Model file for the job. Use its own axes, mm. Face numbers are marked on the shaded views. Round coordinates to 2 decimals unless told otherwise and drop trailing zeros. Write each loop counter-clockwise with the first axis right and the second up, starting at its lowest first coordinate (ties: lowest second). Pieces come first, ordered by that corner, then holes. Notation, with made-up numbers: (48.25, -29) - (89.25, -29) arc R22 cw to (89.25, 8) - close; hole circle Ø8 at (-8, 8). An arc over 180 degrees is marked (long way). Answer as a JSON object with one key per item and string values. Group by question number.
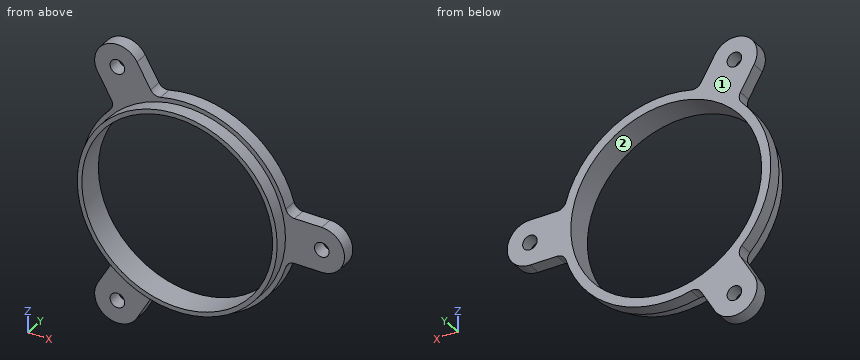
Autodesk Inventor part; units mm, degrees
ref_plane "YZ Plane" through (0, 0, 0) normal (1, 0, 0) x (0, 1, 0)
ref_plane "XZ Plane" through (0, 0, 0) normal (0, 1, 0) x (-1, 0, 0)
ref_plane "XY Plane" through (0, 0, 0) normal (0, 0, 1) x (1, 0, 0)
sketch "Sketch1" plane through (0, 0, 0) normal (0, 0, 1) x (1, 0, 0)
  line L0 (-21, 0) -> (-21, 6)
  line L1 (-21, 6) -> (-23, 6)
  line L2 (-23, 6) -> (-23, 3)
  line L3 (-23, 3) -> (-22, 3)
  line L4 (-22, 3) -> (-22, 0)
  line L5 (-22, 0) -> (-21, 0)
  line L6 (0, -1.2) -> (0, 7.2)
  point P0 (0, 0)
  point P1 (-22, 1.5)
  dimension "d0" = 22
  dimension "d1" = 1
  dimension "d2" = 23
  dimension "d3" = 3
  dimension "d4" = 3
revolve "Revolution1" add sketch "Sketch1" angle 360 about axis through (0, -10, 0) along (0, 1, 0)
sketch "Sketch2" plane through (0, 6, 0) normal (0, 1, 0) x (1, 0, 0)
  circle A0 centre (0, 0) radius 30 construction
  circle A1 centre (30, 0) radius 5
  circle A2 centre (0, 0) radius 23
  line L0 (30, 5) -> (22.4499, 5)
  line L1 (30, -5) -> (22.4499, -5)
  dimension "d6" = 60
  dimension "d7" = 10
extrude "Extrusion1" add sketch "Sketch2" against normal blind 3 contours A1 | A1 L1 A2 L0
fillet "Fillet1" radius 2 2 edges at (22.4499, 4.5, 5) (22.4499, 4.5, -5)
sketch "Sketch3" plane through (30, 6, 0) normal (0, 1, 0) x (1, 0, 0)
  arc A0 (0, -5) -> (0, 5) centre (0, 0) ccw
  point P0 (-30, 0)
hole "Hole1" at (30, 6, 0) direction (0, -1, 0) diameter 3.2 end through all
pattern_circular "Circular Pattern1" count 3 over 360 about axis through (0, 3, 0) along (0, 1, 0) of "Extrusion1", "Hole1", "Fillet1"
properties part number "Electrode-Fixed-Press" material "Brass"
(1) Flat gauge pins, fed straight in: pin 1 (0.9 mm diameter, centred on x = 28.5, y = 4.5, fed in from -Z); pin 2 (1 mm diameter, centred on x = 18.5, y = 3, fed in from +Z); pin 3 (1.5 mm diameter, centred on x = 16, y = 1.5, fed in from +Z); pin 4 (3 mm diameter, centred on x = -15, z = -25.98, fed in from +Y). Where does each tip first touch, or does it go through?
(2) Slice it at D-D (y = 4.9). Write the cut outline in (x, z), then the cut area to 3 significant figures.
(3) Slice it at A-A (x = 0). Write the cut outline in (y, z).
(4) Pull direction X, two halves, no side cores. Call the marked faces 1 and 2: pulls with the +X half, pulls with the -X half, needs draft (parallel to the pull), parting line crosses it, or undercut.
(5) Slice it at B-B (z = 0). Write the cut outline in (x, y), then the cut area to 3 significant figures.
(6) Drill centre lines: line 1 (Z direction, x = 30, y = 5.1); line 2 (X direction, y = 2.2, z = -7.5); line 3 (X direction, y = 0.3, z = 11). Where is each one in solid material? Low to high. Write a range as from..to.
(7) Slice it at C-C (z = 26.5). Write the cut outline in (x, y), then the cut area to 3 significant figures.
Answer:
{
 "1": {"pin 1": "z = -5", "pin 2": "z = 14.32", "pin 3": "z = 15.86", "pin 4": "through"},
 "2": {"outline": "(-19.33, -23.48) arc R5 ccw to (-10.67, -28.48) - (-7.67, -23.28) arc R2 cw to (-5.46, -22.34) arc R23 ccw to (22.08, -6.44) arc R2 cw to (24, -5) - (30, -5) arc R5 ccw to (30, 5) - (24, 5) arc R2 cw to (22.08, 6.44) arc R23 ccw to (-5.46, 22.34) arc R2 cw to (-7.67, 23.28) - (-10.67, 28.48) arc R5 ccw to (-19.33, 23.48) - (-16.33, 18.28) arc R2 cw to (-16.62, 15.9) arc R23 ccw to (-16.62, -15.9) arc R2 cw to (-16.33, -18.28) - close; hole circle Ø42 at (0, 0); hole circle Ø3.2 at (-15, -25.98); hole circle Ø3.2 at (-15, 25.98); hole circle Ø3.2 at (30, 0)", "area": "588 mm²"},
 "3": {"outline": "(0, -22) - (3, -22) - (3, -23) - (6, -23) - (6, -21) - (0, -21) - close; (0, 21) - (6, 21) - (6, 23) - (3, 23) - (3, 22) - (0, 22) - close"},
 "4": {"face 1": "needs draft", "face 2": "undercut"},
 "5": {"outline": "(-23, 3) - (-22, 3) - (-22, 0) - (-21, 0) - (-21, 6) - (-23, 6) - close; (21, 0) - (22, 0) - (22, 3) - (28.4, 3) - (28.4, 6) - (21, 6) - close; (31.6, 3) - (35, 3) - (35, 6) - (31.6, 6) - close", "area": "44.4 mm²"},
 "6": {"line 1": "-5..-1.6, 1.6..5", "line 2": "-20.68..-19.62, 19.62..20.68", "line 3": "-19.05..-17.89, 17.89..19.05"},
 "7": {"outline": "(-19.97, 3) - (-16.51, 3) - (-16.51, 6) - (-19.97, 6) - close; (-13.49, 3) - (-9.53, 3) - (-9.53, 6) - (-13.49, 6) - close", "area": "22.3 mm²"}
}
